Autodesk Inventor part; units mm, degrees
ref_plane "YZ Plane" through (0, 0, 0) normal (1, 0, 0) x (0, 1, 0)
ref_plane "XZ Plane" through (0, 0, 0) normal (0, 1, 0) x (-1, 0, 0)
ref_plane "XY Plane" through (0, 0, 0) normal (0, 0, 1) x (1, 0, 0)
sketch "Esboço1" plane through (0, 0, 0) normal (0, 0, 1) x (1, 0, 0)
  line L0 (0, 0) -> (440, 0)
  line L1 (440, 0) -> (440, 310)
  line L2 (440, 310) -> (0, 310)
  line L3 (0, 310) -> (0, 0)
  line L4 (440, 310) -> (445, 310)
  line L5 (445, 310) -> (445, 0)
  line L6 (445, 0) -> (440, 0)
  line L7 (0, 310) -> (-5, 310)
  line L8 (-5, 310) -> (-5, 0)
  line L9 (-5, 0) -> (0, 0)
  dimension "d0" = 440
  dimension "d1" = 310
  dimension "d2" = 5
  dimension "d3" = 5
extrude "Extrusão1" add sketch "Esboço1" along normal blind 5
extrude "Extrusão2" add sketch "Esboço1" against normal blind 40 contours L9 L8 L7 L3 | L1 L4 L5 L6
properties part number "TesteProteção"
The listing builds one solid part. Answer for the finished solid, in the listing's coordinates (mm). A direction names the side the tool comes from. Coordinates: 2 decimals unless noted, no trailing zeros. Write each loop counter-clockwise with the first axis right and the second up, starting at its lowest first coordinate (ties: lowest second). Pieces come first, ordered by that corner, then holes.
Q1. Section A-A, the plane z = -29.5 is taken. Write down the section's boundary in (x, y), then the cut area to 3 significant figures.
Returned:
outline: (-5, 0) - (0, 0) - (0, 310) - (-5, 310) - close; (440, 0) - (445, 0) - (445, 310) - (440, 310) - close
area: 3,100 mm2
Q2. Given P1, Ø4, axis at x = 130.5, y = 183.5, coming from the -Z side, flat-ended and moving along its own axis, determine where the tip first touches the part or whether it passes through.
Returned:
P1: stops at z = 0
Q3. Section B-B, the plane y = 265 is taken. Write down the section's boundary in (x, z).
Returned:
outline: (-5, -40) - (0, -40) - (0, 0) - (440, 0) - (440, -40) - (445, -40) - (445, 5) - (-5, 5) - close
Q4. Find the intervals of material crossed by line 1 along X through (y, z) = (216.5, -28); line 2 along Z through (x, y) = (39.5, 197), in increasing order.
Returned:
line 1: x = -5 to 0, 440 to 445
line 2: z = 0 to 5
Q5. The mould has two halves that part along X. Classify faces 3 (the flat face through (-5, 157, -18)), 4 (the flat face through (445, 157, -18)), 5 (the flat face through (221, 310, 2)), 6 (the flat face through (440, 153, -20)): released by +X, released by -X, zero draft, split by the parting line, or undercut.
Returned:
face 3: released by -X
face 4: released by +X
face 5: zero draft
face 6: undercut
Q6. Section C-C, the plane x = 182.5 is taken. Write down the section's boundary in (y, z), then the cut area to 3 significant figures.
Returned:
outline: (0, 0) - (310, 0) - (310, 5) - (0, 5) - close
area: 1,550 mm2
Q7. Which of the six approach directions +Z, -Z, +X, -X, +Y, -Y give full straight-line access (tool end or side, diameter ignored) to faces 1 (the flat face through (217, 157, 0)), 2 (the flat face through (217, 157, 5))?
Returned:
face 1: -Z, +Y, -Y
face 2: +Z, +X, -X, +Y, -Y
